```python
from build123d import *

# Parameters (mm, degrees)
SKETCH12_W         = 6.35
SKETCH12_H         = 1.7526
CHAMFER1_SIZE      = 0.5953125
CUT_EXTRUDE2_DEPTH = 1.72466


with BuildPart() as part:
    # Sketch12 → Revolve3 (revolve)
    with BuildSketch(Plane(origin=(0, 0, 0), x_dir=(0, 0, -1), z_dir=(1, 0, 0))):
        with Locations((0, 0.8763)):
            Rectangle(SKETCH12_W, SKETCH12_H)
    revolve(axis=Axis((0, 0, -3.175), (0, 0, 1)))

    # Sketch7 → Revolve2 (revolve)
    with BuildSketch(Plane(origin=(0, 0, 0), x_dir=(0, 0, -1), z_dir=(1, 0, 0)), mode=Mode.PRIVATE) as revolve2_sk:
        with BuildLine():
            Line((-3.175, 3.8989), (-2.92862, 3.8989))
            Line((-2.92862, 3.8989), (-0.7112, 1.971326202))
            ThreePointArc((-0.7112, 1.971326202), (-0.43847117, 1.809069598), (-0.126190199, 1.7526))
            Line((-0.126190199, 1.7526), (-0.126190199, 0))
            Line((-0.126190199, 0), (-3.175, 0))
            Line((-3.175, 0), (-3.175, 3.8989))
        make_face()
    revolve(revolve2_sk.sketch.rotate(Axis((0, 0, 3.175), (0, 0, -1)), 180), axis=Axis((0, 0, 3.175), (0, 0, -1)))

    # Chamfer1
    chamfer1_edges = [part.edges().sort_by_distance(p)[0] for p in [
        (0, -1.7526, -3.175),
    ]]
    chamfer(chamfer1_edges, length=CHAMFER1_SIZE)

    # Sketch5 → Cut-Extrude2 (cut)
    with BuildSketch(Plane.XY.offset(3.175)):
        Polygon((0, 1.14567944), (-0.9921875, 0.57283972), (-0.9921875, -0.57283972), (0, -1.14567944), (0.9921875, -0.57283972), (0.9921875, 0.57283972), align=None)
    extrude(amount=-CUT_EXTRUDE2_DEPTH, mode=Mode.SUBTRACT)

    # Cut-Extrude3 cone 1 section (on through the dimple's axis) → Cut-Extrude3 (revolve, cut)
    with BuildSketch(Plane(origin=(0, 0, 3.175), x_dir=(0, -1, 0), z_dir=(1, 0, 0))):
        Polygon((0, 0), (1.14567944, 0), (0, 1.14567944), align=None)
    revolve(axis=Axis((0, 0, 3.175), (0, 0, -1)), mode=Mode.SUBTRACT)


solid = part.part
```
The listing builds one solid part. Answer for the finished solid, in the listing's coordinates (mm). A direction names the side the tool comes from. Round coordinates to 2 decimals unless told otherwise and drop trailing zeros. Order: outer loops, then holes, each group sorted by start corner. A loop starts at its lowest first (then second) coordinate and runs counter-clockwise, first axis right, second up. Notation, with made-up numbers: (-14.75, 14.5) - (23.25, 14.5) arc R33 ccw to (23.25, 46.5) - close; hole circle Ø10 at (-31, 86.25). An arc over 180 degrees is marked (long way). Put each result on its own line as item: value. Start each with the question number.
(1) Find section C-C (z = 2.5). Give the vertices of the cut face in (x, y), plus the area to 3 significant figures.
(2) Determine the mould class of faces 3 (the cylindrical face through (-0.53, 1.67, -1.25)), 4 (the flat face through (0, 0, -3.175)), 5 (the flat face through (0.489, -0.863, 2.325)), 6 (the flat face through (-0.503, -0.855, 2.325)) for opening direction Y: released by +Y, released by -Y, zero draft, split by the parting line, or undercut.
(3) For faces 1 (the flat face through (-0.992, 0, 2)), 2 (the flat face through (1, 1, 3.175)), determine the directions among +Z, -Z, +X, -X, +Y, -Y from which every point of the face is accessible in a straight line to the end or side of a thin tool.
(4) Find section D-D (z = 0.25). Give the vertices of the cut face in (x, y), plus the area to 3 significant figures.
(5) Find section B-B (z = -1). Give the vertices of the cut face in (x, y).
(6) Straight lines are drawn through the part: probe 1 along X at (y, z) = (-0.25, 3); probe 2 along X at (y, z) = (0, 1.5); probe 3 along Z at (x, y) = (3.25, 0) (3 decimals). For each, find the intervals that lie inside material, in ascending order. Write a range as from..to.
(7) Given P1, Ø1.3, axis at y = 0, z = 2, coming from the +X side; P2, Ø4, axis at x = -3, y = 2.5, coming from the -Z side; P3, Ø0.9, axis at y = 0, z = 2, coming from the -X side; P4, Ø3, axis at x = -0.5, z = 2.5, coming from the +Y side, each flat-ended and moving along its own axis, determine where each tip first touches the part or whether it passes through.
Reply:
1. outline: circle Ø7.05 at (0, 0); hole (-0.99, -0.57) - (0, -1.15) - (0.99, -0.57) - (0.99, 0.57) - (0, 1.15) - (-0.99, 0.57) - close
1. area: 35.7 mm^2
2. face 3: split by the parting line
2. face 4: zero draft
2. face 5: undercut
2. face 6: undercut
3. face 1: +Z
3. face 2: +Z, +X, -X, +Y, -Y
4. outline: circle Ø3.52 at (0, 0)
4. area: 9.75 mm^2
5. outline: circle Ø3.51 at (0, 0)
6. probe 1: -3.89..-0.99, 0.99..3.89
6. probe 2: -2.66..-0.99, 0.99..2.66
6. probe 3: 2.182..3.175
7. P1: x = 3.66
7. P2: z = 0.62
7. P3: x = -3.48
7. P4: y = 3.9
